```python
from build123d import *

# Parameters (mm, degrees)
EPIFISIS_DISTAL_DEPTH    = 18
OREJA_MEDIAL_DEPTH       = 4
OREJA_LATERAL_DEPTH      = 4
SKETCH4_R                = 2.6
AGUJERO_EJE_MUNECA_DEPTH = 1000


with BuildPart() as part:
    # Sketch1 → Epifisis_distal (new body)
    with BuildSketch(Plane.XY.offset(-9)):
        Polygon((-7.5, 52), (18, 52), (20.5, 30), (19.5, 15), (-19.5, 15), (-19.5, 17.5), (-7.5, 17.5), align=None)
    extrude(amount=EPIFISIS_DISTAL_DEPTH)

    # Sketch2 → Oreja_medial (add)
    with BuildSketch(Plane(origin=(-19.5, 0, 0), x_dir=(0, 0, -1), z_dir=(1, 0, 0))):
        with BuildLine():
            Line((8, 15), (8, 0))
            ThreePointArc((8, 0), (0, -8), (-8, 0))
            Line((-8, 0), (-8, 15))
            ThreePointArc((-8, 15), (0, 23), (8, 15))
        make_face()
    extrude(amount=OREJA_MEDIAL_DEPTH)

    # Sketch3 → Oreja_lateral (add)
    with BuildSketch(Plane(origin=(15.5, 0, 0), x_dir=(0, 0, -1), z_dir=(1, 0, 0))):
        with BuildLine():
            Line((8, 15), (8, 0))
            ThreePointArc((8, 0), (0, -8), (-8, 0))
            Line((-8, 0), (-8, 15))
            ThreePointArc((-8, 15), (0, 23), (8, 15))
        make_face()
    extrude(amount=OREJA_LATERAL_DEPTH)

    # Sketch4 → Agujero_eje_muneca (cut, symmetric)
    with BuildSketch(Plane(origin=(0, 0, 0), x_dir=(0, 0, -1), z_dir=(1, 0, 0))):
        Circle(SKETCH4_R)
    extrude(amount=AGUJERO_EJE_MUNECA_DEPTH, both=True, mode=Mode.SUBTRACT)


solid = part.part
```
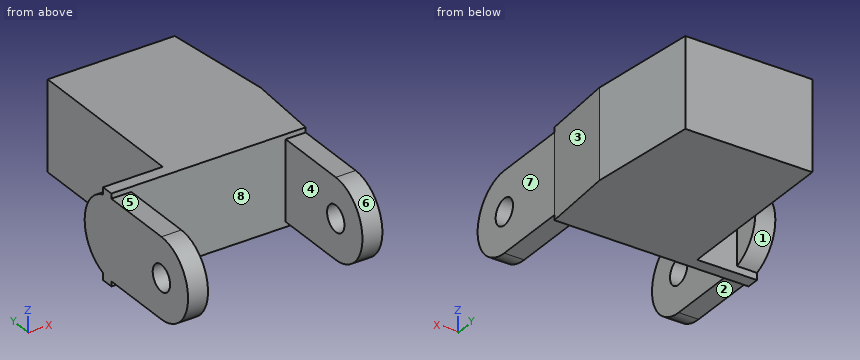
Verification items for the finished model (mm, model axes). Face numbers are marked on the shaded views. A direction names the side the tool comes from. Round coordinates to 2 decimals unless told otherwise and drop trailing zeros. Order: outer loops, then holes, each group sorted by start corner. A loop starts at its lowest first (then second) coordinate and runs counter-clockwise, first axis right, second up. Notation, with made-up numbers: (11.5, -37.75) - (35.5, -37.75) arc R20 cw to (35.5, -27.75) - close; hole circle Ø8 at (36, 61). An arc over 180 degrees is marked (long way). Use CSV: the item, a comma, the result in double quotes. Start each with the question number.
1) Access from +Z, -Z, +X, -X, +Y, -Y to the whole of each face (thin tool, end or side, straight path). Record for the marked faces 1, 2, 3, 4 and 5.
2) Section check B-B, the plane z = 0. Record the cut outline in (x, y).
3) Mould release check, pull along X, two halves, no side actions. Record for the marked faces 6, 7 and 8: +X half, -X half, draft (parallel to the pull), parting line (faces both ways), or undercut.
4) Section check A-A, the plane y = 4. Record the cut outline in (x, z).
5) Thickness scan on L1, parallel to X at y = 0.5, z = -7; L2, parallel to Y at x = -17, z = 0.25; L3, parallel to Y at x = 17.25, z = 0. Record the ranges inside material, lowest first.
6) Section check D-D, the plane y = 38.5. Record the cut outline in (x, z), plus the area to 3 significant figures.
7) Section check C-C, the plane z = 4.5. Record the cut outline in (x, y).
8) Go/stop test with flat-tipped pins: P1, Ø3, axis at x = -17.5, y = 11, coming from the +Z side; P2, Ø5, axis at y = 8, z = 3, coming from the +X side; P3, Ø1.5, axis at x = 14.5, z = -3.5, coming from the -Y side. Record where each tip stops, or that it passes through.
Answers:
1,face 1,"-X, +Y"
1,face 2,"-Z, +X, -X, -Y"
1,face 3,"+Z, -Z, +X, -Y"
1,face 4,"+Z, -Z, -Y"
1,face 5,"+Z, +X, -X, -Y"
2,outline,"(-19.5, -8) - (-15.5, -8) - (-15.5, -2.6) - (-19.5, -2.6) - close; (-19.5, 2.6) - (-15.5, 2.6) - (-15.5, 15) - (15.5, 15) - (15.5, 2.6) - (19.5, 2.6) - (19.5, 15) - (20.5, 30) - (18, 52) - (-7.5, 52) - (-7.5, 17.5) - (-15.5, 17.5) - (-15.5, 23) - (-19.5, 23) - close; (15.5, -8) - (19.5, -8) - (19.5, -2.6) - (15.5, -2.6) - close"
3,face 6,"draft"
3,face 7,"+X half"
3,face 8,"undercut"
4,outline,"(-19.5, -8) - (-15.5, -8) - (-15.5, 8) - (-19.5, 8) - close; (15.5, -8) - (19.5, -8) - (19.5, 8) - (15.5, 8) - close"
5,L1,"x = -19.5 to -15.5, 15.5 to 19.5"
5,L2,"y = -8 to -2.59, 2.59 to 23"
5,L3,"y = -8 to -2.6, 2.6 to 52"
6,outline,"(-7.5, -9) - (19.53, -9) - (19.53, 9) - (-7.5, 9) - close"
6,area,"487 mm²"
7,outline,"(-19.5, -6.61) - (-15.5, -6.61) - (-15.5, 15) - (15.5, 15) - (15.5, -6.61) - (19.5, -6.61) - (19.5, 15) - (20.5, 30) - (18, 52) - (-7.5, 52) - (-7.5, 17.5) - (-15.5, 17.5) - (-15.5, 21.61) - (-19.5, 21.61) - close"
8,P1,"stops at z = 8"
8,P2,"stops at x = 19.5"
8,P3,"stops at y = 15"
